Input: part model. Units: mm. Frame: model coordinates. A direction names the side the tool comes from. Give positions to 0.01 mm unless a question says otherwise; leave off trailing zeros. Write each loop counter-clockwise with the first axis right and the second up, starting at its lowest first coordinate (ties: lowest second). Pieces come first, ordered by that corner, then holes.
```python
from build123d import *

# Parameters (mm, degrees)
F0_W      = 65
F0_H      = 45
F1_DEPTH  = 3
F3_DEPTH  = 4.5
F4_R      = 1.5
F5_DEPTH  = 25
F7_DEPTH  = 2
F9_DEPTH  = 4
F11_DEPTH = 3
F13_DEPTH = 2
F15_DEPTH = 1


with BuildPart() as f1:
    # F0 (on Front) → F1 (new body)
    with BuildSketch(Plane.XZ):
        Rectangle(F0_W, F0_H)
    extrude(amount=F1_DEPTH)

    # F2 (on face) → F3 (join)
    with BuildSketch(Plane.XZ.offset(3)):
        with BuildLine():
            Line((22.085, 18.985), (-22.085, 18.985))
            ThreePointArc((-22.085, 18.985), (-24.13561, 18.13561), (-24.985, 16.085))
            Line((-24.985, 16.085), (-24.985, -16.085))
            ThreePointArc((-24.985, -16.085), (-24.13561, -18.13561), (-22.085, -18.985))
            Line((-22.085, -18.985), (22.085, -18.985))
            ThreePointArc((22.085, -18.985), (24.13561, -18.13561), (24.985, -16.085))
            Line((24.985, -16.085), (24.985, 16.085))
            ThreePointArc((24.985, 16.085), (24.13561, 18.13561), (22.085, 18.985))
        make_face()
    extrude(amount=F3_DEPTH)

    # F4 (on face) → F5 (cut)
    with BuildSketch(Plane.XZ.offset(7.5)):
        with BuildLine():
            Line((9.6, 11.4), (-9.6, 11.4))
            ThreePointArc((-9.6, 11.4), (-11.72132, 10.52132), (-12.6, 8.4))
            Line((-12.6, 8.4), (-12.6, -8.4))
            ThreePointArc((-12.6, -8.4), (-11.72132, -10.52132), (-9.6, -11.4))
            Line((-9.6, -11.4), (9.6, -11.4))
            ThreePointArc((9.6, -11.4), (11.72132, -10.52132), (12.6, -8.4))
            Line((12.6, -8.4), (12.6, 8.4))
            ThreePointArc((12.6, 8.4), (11.72132, 10.52132), (9.6, 11.4))
        make_face()
        with Locations((-29, 0)):
            Circle(F4_R)
        with Locations((29, 0)):
            Circle(F4_R)
    extrude(amount=-F5_DEPTH, mode=Mode.SUBTRACT)

    # F6 (on face) → F7 (cut)
    with BuildSketch(Plane(origin=(0, 0, 0), x_dir=(-1, 0, 0), z_dir=(0, 1, 0))):
        with BuildLine():
            Line((-18.3, -12.8), (-21.9, -12.8))
            ThreePointArc((-21.9, -12.8), (-22.607107, -13.092893), (-22.9, -13.8))
            Line((-22.9, -13.8), (-22.9, -16.25))
            ThreePointArc((-22.9, -16.25), (-22.607107, -16.957107), (-21.9, -17.25))
            Line((-21.9, -17.25), (25.1, -17.25))
            ThreePointArc((25.1, -17.25), (25.807107, -16.957107), (26.1, -16.25))
            Line((26.1, -16.25), (26.1, -13.8))
            ThreePointArc((26.1, -13.8), (25.807107, -13.092893), (25.1, -12.8))
            Line((25.1, -12.8), (21.5, -12.8))
            ThreePointArc((21.5, -12.8), (21.287868, -12.712132), (21.2, -12.5))
            Line((21.2, -12.5), (21.2, -9.3))
            ThreePointArc((21.2, -9.3), (21.287868, -9.087868), (21.5, -9))
            Line((21.5, -9), (25.1, -9))
            ThreePointArc((25.1, -9), (25.807107, -8.707107), (26.1, -8))
            Line((26.1, -8), (26.1, 8))
            ThreePointArc((26.1, 8), (25.807107, 8.707107), (25.1, 9))
            Line((25.1, 9), (21.5, 9))
            ThreePointArc((21.5, 9), (21.287868, 9.087868), (21.2, 9.3))
            Line((21.2, 9.3), (21.2, 12.5))
            ThreePointArc((21.2, 12.5), (21.287868, 12.712132), (21.5, 12.8))
            Line((21.5, 12.8), (25.1, 12.8))
            ThreePointArc((25.1, 12.8), (25.807107, 13.092893), (26.1, 13.8))
            Line((26.1, 13.8), (26.1, 16.25))
            ThreePointArc((26.1, 16.25), (25.807107, 16.957107), (25.1, 17.25))
            Line((25.1, 17.25), (-21.9, 17.25))
            ThreePointArc((-21.9, 17.25), (-22.607107, 16.957107), (-22.9, 16.25))
            Line((-22.9, 16.25), (-22.9, 13.8))
            ThreePointArc((-22.9, 13.8), (-22.607107, 13.092893), (-21.9, 12.8))
            Line((-21.9, 12.8), (-18.3, 12.8))
            ThreePointArc((-18.3, 12.8), (-18.087868, 12.712132), (-18, 12.5))
            Line((-18, 12.5), (-18, 9.3))
            ThreePointArc((-18, 9.3), (-18.087868, 9.087868), (-18.3, 9))
            Line((-18.3, 9), (-21.9, 9))
            ThreePointArc((-21.9, 9), (-22.607107, 8.707107), (-22.9, 8))
            Line((-22.9, 8), (-22.9, -8))
            ThreePointArc((-22.9, -8), (-22.607107, -8.707107), (-21.9, -9))
            Line((-21.9, -9), (-18.3, -9))
            ThreePointArc((-18.3, -9), (-18.087868, -9.087868), (-18, -9.3))
            Line((-18, -9.3), (-18, -12.5))
            ThreePointArc((-18, -12.5), (-18.087868, -12.712132), (-18.3, -12.8))
        make_face()
    extrude(amount=-F7_DEPTH, mode=Mode.SUBTRACT)

    # F8 (on face) → F9 (cut)
    with BuildSketch(Plane.XZ.offset(7.5)):
        with BuildLine():
            Line((9.6, 12.4), (-9.6, 12.4))
            ThreePointArc((-9.6, 12.4), (-12.428427, 11.228427), (-13.6, 8.4))
            Line((-13.6, 8.4), (-13.6, -8.4))
            ThreePointArc((-13.6, -8.4), (-12.428427, -11.228427), (-9.6, -12.4))
            Line((-9.6, -12.4), (9.6, -12.4))
            ThreePointArc((9.6, -12.4), (12.428427, -11.228427), (13.6, -8.4))
            Line((13.6, -8.4), (13.6, 8.4))
            ThreePointArc((13.6, 8.4), (12.428427, 11.228427), (9.6, 12.4))
        make_face()
    extrude(amount=-F9_DEPTH, mode=Mode.SUBTRACT)

    # F10 (on face) → F11 (cut)
    with BuildSketch(Plane.XZ.offset(7.5)):
        with BuildLine():
            Line((9.6, 13.4), (-9.6, 13.4))
            ThreePointArc((-9.6, 13.4), (-13.135534, 11.935534), (-14.6, 8.4))
            Line((-14.6, 8.4), (-14.6, -8.4))
            ThreePointArc((-14.6, -8.4), (-13.135534, -11.935534), (-9.6, -13.4))
            Line((-9.6, -13.4), (9.6, -13.4))
            ThreePointArc((9.6, -13.4), (13.135534, -11.935534), (14.6, -8.4))
            Line((14.6, -8.4), (14.6, 8.4))
            ThreePointArc((14.6, 8.4), (13.135534, 11.935534), (9.6, 13.4))
        make_face()
    extrude(amount=-F11_DEPTH, mode=Mode.SUBTRACT)

    # F12 (on face) → F13 (cut)
    with BuildSketch(Plane.XZ.offset(7.5)):
        with BuildLine():
            Line((9.6, 14.4), (-9.6, 14.4))
            ThreePointArc((-9.6, 14.4), (-13.842641, 12.642641), (-15.6, 8.4))
            Line((-15.6, 8.4), (-15.6, -8.4))
            ThreePointArc((-15.6, -8.4), (-13.842641, -12.642641), (-9.6, -14.4))
            Line((-9.6, -14.4), (9.6, -14.4))
            ThreePointArc((9.6, -14.4), (13.842641, -12.642641), (15.6, -8.4))
            Line((15.6, -8.4), (15.6, 8.4))
            ThreePointArc((15.6, 8.4), (13.842641, 12.642641), (9.6, 14.4))
        make_face()
    extrude(amount=-F13_DEPTH, mode=Mode.SUBTRACT)

    # F14 (on face) → F15 (cut)
    with BuildSketch(Plane.XZ.offset(7.5)):
        with BuildLine():
            Line((9.6, 15.4), (-9.6, 15.4))
            ThreePointArc((-9.6, 15.4), (-11.825421, 15.036829), (-13.819926, 13.985))
            Line((-13.819926, 13.985), (13.819926, 13.985))
            ThreePointArc((13.819926, 13.985), (11.825421, 15.036829), (9.6, 15.4))
        make_face()
        with BuildLine():
            Line((13.819926, -13.985), (-13.819926, -13.985))
            ThreePointArc((-13.819926, -13.985), (-11.825421, -15.036829), (-9.6, -15.4))
            Line((-9.6, -15.4), (9.6, -15.4))
            ThreePointArc((9.6, -15.4), (11.825421, -15.036829), (13.819926, -13.985))
        make_face()
        with BuildLine():
            Line((13.819926, 13.985), (-13.819926, 13.985))
            ThreePointArc((-13.819926, 13.985), (-15.866557, 11.519336), (-16.6, 8.4))
            Line((-16.6, 8.4), (-16.6, -8.4))
            ThreePointArc((-16.6, -8.4), (-15.866557, -11.519336), (-13.819926, -13.985))
            Line((-13.819926, -13.985), (13.819926, -13.985))
            ThreePointArc((13.819926, -13.985), (15.866557, -11.519336), (16.6, -8.4))
            Line((16.6, -8.4), (16.6, 8.4))
            ThreePointArc((16.6, 8.4), (15.866557, 11.519336), (13.819926, 13.985))
        make_face()
    extrude(amount=-F15_DEPTH, mode=Mode.SUBTRACT)


solid = f1.part
```
Q1. Access query for faces 1 (the cylindrical face through (-13.1, -5.01, 11.97)), 2 (the flat face through (-26.1, -1, 15)), 3 (the flat face through (24.985, -5, 0)), 4 (the cylindrical face through (11.74, -2.76, 10.5)). Directions: +Z, -Z, +X, -X, +Y, -Y. A direction counts if a zero-diameter tool reaches every point of the face in a straight line with its end or side. Return the directions, or none.
Q2. Material intervals for line 1 along X through (y, z) = (-1, 11.5); line 2 along Z through (x, y) = (29, -2.3); line 3 along X through (y, z) = (-5.75, 5) (3 decimals), sorted ascending.
Q3. Section D-D, the plane z = 18. Return the cut outline in (x, y).
Q4. Section A-A, the plane x = -29. Return the cut outline in (y, z), then the cut area to 3 significant figures.
Q5. Mould query, pull axis X, two halves, no side actions, for faces 5 (the flat face through (0, -3, 11.4)), 6 (the flat face through (-32.5, -1, 0)), 7 (the flat face through (32.5, -1, 0)), 8 (the flat face through (12.6, -3, 0)). Classes: +X half, -X half, draft (parallel to the pull), parting line (faces both ways), or undercut.
Q6. Pin query (flat end, axial travel): pin 1 (1.5 mm diameter, centred on x = 11, y = -4, fed in from -Z) (3 decimals); pin 2 (12 mm diameter, centred on x = 8.5, z = 5.5, fed in from +Y). Return the tip coordinate at first contact, or that it passes through.
Solutions:
1. face 1: -Y
1. face 2: +Y
1. face 3: +Z, -Z, +X, -Y
1. face 4: +Y, -Y
2. line 1: x = -32.5 to -21.2, 18 to 32.5
2. line 2: z = -22.5 to -1.5, 1.5 to 22.5
2. line 3: x = -24.985 to -15.6, 15.6 to 24.985
3. outline: (-32.5, -3) - (-24.26, -3) - (-24.26, -7.5) - (24.26, -7.5) - (24.26, -3) - (32.5, -3) - (32.5, 0) - (-32.5, 0) - close
4. outline: (-3, -22.5) - (0, -22.5) - (0, -1.5) - (-3, -1.5) - close; (-3, 1.5) - (0, 1.5) - (0, 22.5) - (-3, 22.5) - close
4. area: 126 mm2
5. face 5: undercut
5. face 6: -X half
5. face 7: +X half
5. face 8: undercut
6. pin 1: stops at z = -18.985
6. pin 2: stops at y = -2
